Source: CAD feature listing. Evaluate the final solid. Frame: model axes, mm. Face numbers are marked on the shaded views. Give positions to 0.01 mm unless a question says otherwise; leave off trailing zeros. Order: outer loops, then holes, each group sorted by start corner. A loop starts at its lowest first (then second) coordinate and runs counter-clockwise, first axis right, second up.
```python
from build123d import *

# Parameters (mm, degrees)
CYLINDER_R          = 16.7005
CYLINDER_DEPTH      = 476.25
CYLINDER_ROLL_ANGLE = 90
THICKNESS001_T      = -3.3782


with BuildPart() as part:
    # Cylinder → Cylinder (new body)
    with BuildSketch(Plane.XY):
        Circle(CYLINDER_R)
    extrude(amount=CYLINDER_DEPTH)


with BuildPart() as part_1:
    # Cylinder roll: moved
    add(part.part.rotate(Axis((0, 0, 0), (1, 0, 0)), CYLINDER_ROLL_ANGLE))


with BuildPart() as part_2:
    # Cylinder placement: moved
    add(part_1.part)

    # Thickness001
    thickness001_openings = [part_2.faces().sort_by_distance(p)[0] for p in [
        (0, 0, 0),
        (0, -476.25, 0),
    ]]
    offset(amount=THICKNESS001_T, openings=thickness001_openings)


solid = part_2.part
```
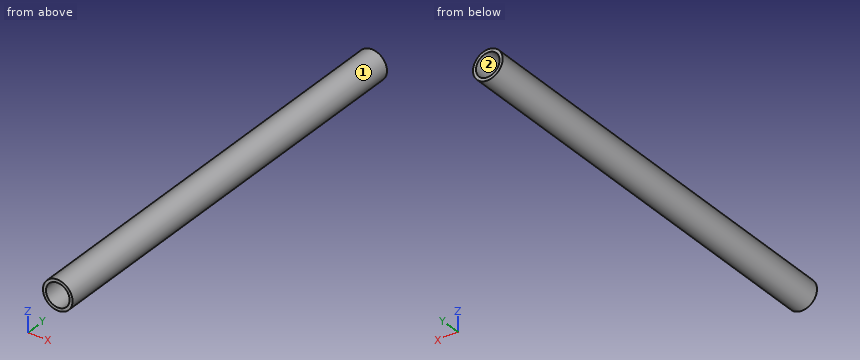
1) Section query B-B, the plane z = 0. Return the cut outline in (x, y).
Report:
outline: (-16.7, -476.25) - (-13.32, -476.25) - (-13.32, 0) - (-16.7, 0) - close; (13.32, -476.25) - (16.7, -476.25) - (16.7, 0) - (13.32, 0) - close
2) Section query C-C, the plane y = -295. Return the cut outline in (x, z).
Report:
outline: circle Ø33.4 at (0, 0); hole circle Ø26.64 at (0, 0)
3) Section query A-A, the plane x = 0. Return the cut outline in (y, z).
Report:
outline: (-476.25, -16.7) - (0, -16.7) - (0, -13.32) - (-476.25, -13.32) - close; (-476.25, 13.32) - (0, 13.32) - (0, 16.7) - (-476.25, 16.7) - close
4) Draft query along X for the marked faces 1 and 2. Return one class per face: +X half, -X half, draft (parallel to the pull), parting line (faces both ways), or undercut.
Report:
face 1: parting line
face 2: undercut
5) Material intervals for L1, parallel to Z at x = 0, y = -226; L2, parallel to X at y = -325.5, z = 5; L3, parallel to Z at x = 4.5, y = -171.5, sorted ascending.
Report:
L1: z = -16.7 to -13.32, 13.32 to 16.7
L2: x = -15.93 to -12.35, 12.35 to 15.93
L3: z = -16.08 to -12.54, 12.54 to 16.08
6) Pin query (flat end, axial travel): pin 1 (8 mm diameter, centred on x = 9.5, y = -75, fed in from -Z); pin 2 (4 mm diameter, centred on x = -11, y = -347, fed in from -Z); pin 3 (8 mm diameter, centred on x = -13, z = 11.5, fed in from +Y); pin 4 (8 mm diameter, centred on x = 10.5, y = -412, fed in from +Z). Return the tip coordinate at first contact, or that it passes through.
Report:
pin 1: stops at z = -15.77
pin 2: stops at z = -14.07
pin 3: stops at y = 0
pin 4: stops at z = 15.38
